Design review of the part shown in the three views and the two pictorial views. Dimensions are in mm from the part's minimum x, y and z. Give positions to 0.01 mm unless a question says otherwise; leave off trailing zeros. Write each loop counter-clockwise with the first axis right and the second up, starting at its lowest first coordinate (ties: lowest second). Pieces come first, ordered by that corner, then holes. Notation, with made-up numbers: M 80,64 L 92,64 A23 cw 92,81 Z; hole C 18.25,-19 d5. An arc over 180 degrees is marked long. Write item = value, one per line.
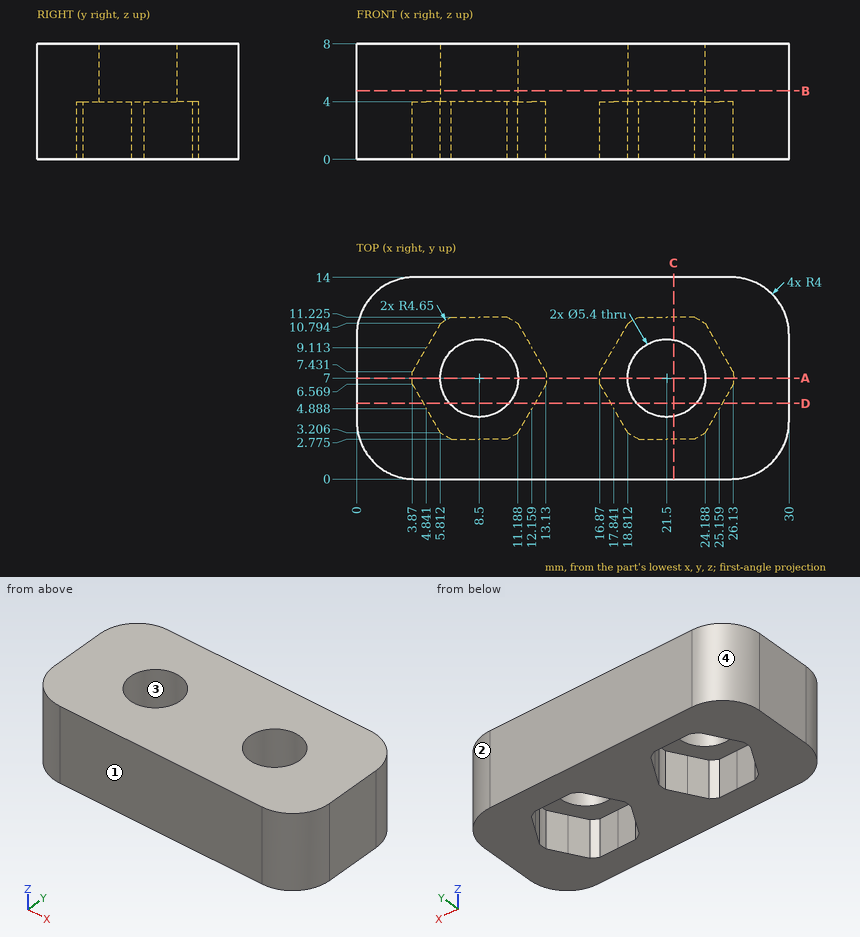
1. We need section B-B, the plane z = 4.75. Write out the cut boundary in (x, y).
Responses:
outline = M 0,4 A4 ccw 4,0 L 26,0 A4 ccw 30,4 L 30,10 A4 ccw 26,14 L 4,14 A4 ccw 0,10 Z; hole C 8.5,7 d5.4; hole C 21.5,7 d5.4
2. The part is to be moulded in two halves that separate along X. For the marked faces 1, 2, 3 and 4, say which applies: +X half, -X half, draft (parallel to the pull), parting line (faces both ways), or undercut.
Responses:
face_1 = draft
face_2 = +X half
face_3 = undercut
face_4 = -X half
3. For line 1 along X through (y, z) = (7, 5.7); line 2 along Y through (x, z) = (8.5, 6.45); line 3 along Y through (x, z) = (9, 1) (1 decimal), list the stretches that pass through material, from the lowest coordinate up. Write a range as from..to.
Responses:
line_1 = 0..5.8, 11.2..18.8, 24.2..30
line_2 = 0..4.3, 9.7..14
line_3 = 0..2.8, 11.2..14
4. Insertion check: P1, Ø7, axis at x = 8.5, y = 7.5, coming from the -Z side. The pin has a flat end and moves straight along its axis. Give the tip position at first contact, or say it passes through.
Responses:
P1 = 4
5. We need section C-C, the plane x = 22. Write out the cut boundary in (y, z) (1 decimal).
Responses:
outline = M 0,0 L 2.8,0 L 2.8,4 L 4.3,4 L 4.3,8 L 0,8 Z; M 9.7,4 L 11.2,4 L 11.2,0 L 14,0 L 14,8 L 9.7,8 Z
6. We need section D-D, the plane y = 5.25. Write out the cut boundary in (x, z).
Responses:
outline = M 0,0 L 4.63,0 L 4.63,4 L 6.44,4 L 6.44,8 L 0,8 Z; M 10.56,4 L 12.37,4 L 12.37,0 L 17.63,0 L 17.63,4 L 19.44,4 L 19.44,8 L 10.56,8 Z; M 23.56,4 L 25.37,4 L 25.37,0 L 30,0 L 30,8 L 23.56,8 Z
7. We need section A-A, the plane y = 7. Write out the cut boundary in (x, z).
Responses:
outline = M 0,0 L 3.85,0 L 3.85,4 L 5.8,4 L 5.8,8 L 0,8 Z; M 11.2,4 L 13.15,4 L 13.15,0 L 16.85,0 L 16.85,4 L 18.8,4 L 18.8,8 L 11.2,8 Z; M 24.2,4 L 26.15,4 L 26.15,0 L 30,0 L 30,8 L 24.2,8 Z
